For this review, use the dimensioned drawing (mm, ordinates from the lowest corner) and the shaded views. Give positions to 0.01 mm unless a question says otherwise; leave off trailing zeros. Order: outer loops, then holes, each group sorted by start corner. A loop starts at its lowest first (then second) coordinate and runs counter-clockwise, first axis right, second up. Notation, with made-up numbers: (65.5, -32.75) - (90.5, -32.75) arc R32 ccw to (90.5, 2.25) - close; hole circle Ø2 at (47.5, -10.5). An arc over 180 degrees is marked (long way). One line per item, written item: value.
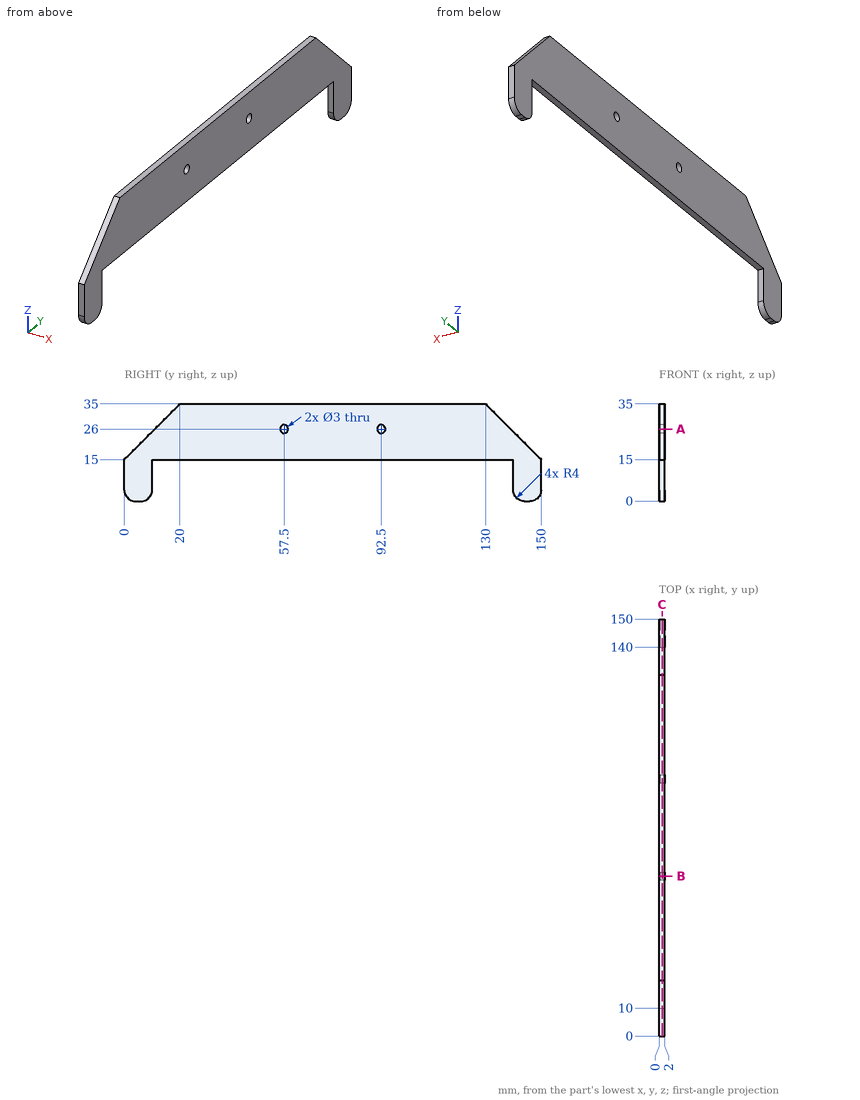
(1) Take a section at C-C (x = 1.1). Write out the cut boundary in (y, z).
Answers below:
outline: (0, 4) arc R4 ccw to (4, 0) - (6, 0) arc R4 ccw to (10, 4) - (10, 15) - (140, 15) - (140, 4) arc R4 ccw to (144, 0) - (146, 0) arc R4 ccw to (150, 4) - (150, 15) - (130, 35) - (20, 35) - (0, 15) - close; hole circle Ø3 at (57.5, 26); hole circle Ø3 at (92.5, 26)
(2) Take a section at B-B (y = 57.5). Write out the cut boundary in (x, z), then the cut area to 3 significant figures.
Answers below:
outline: (0, 15) - (2, 15) - (2, 24.5) - (0, 24.5) - close; (0, 27.5) - (2, 27.5) - (2, 35) - (0, 35) - close
area: 34.0 mm^2
(3) For P1, Ø1, axis at x = 0.5, y = 44.5, coming from the -Z side; P2, Ø10, axis at y = 124, z = 21, coming from the -X side, all flat-tipped, find the tip position at first contact; note any pin that passes through.
Answers below:
P1: stops at z = 15
P2: stops at x = 0
(4) Take a section at A-A (z = 26). Write out the cut boundary in (x, y).
Answers below:
outline: (0, 11) - (2, 11) - (2, 56) - (0, 56) - close; (0, 59) - (2, 59) - (2, 91) - (0, 91) - close; (0, 94) - (2, 94) - (2, 139) - (0, 139) - close
(5) Wall thickness on line 1 (Z direction, x = 1.4, y = 57.5); line 2 (Y direction, x = 1.6, z = 5.5); line 3 (Y direction, x = 0.6, z = 27): over which ranges is each line inside the solid? List them lowest first. Write a range as from..to.
Answers below:
line 1: z = 15..24.5, 27.5..35
line 2: y = 0..10, 140..150
line 3: y = 12..56.38, 58.62..91.38, 93.62..138
